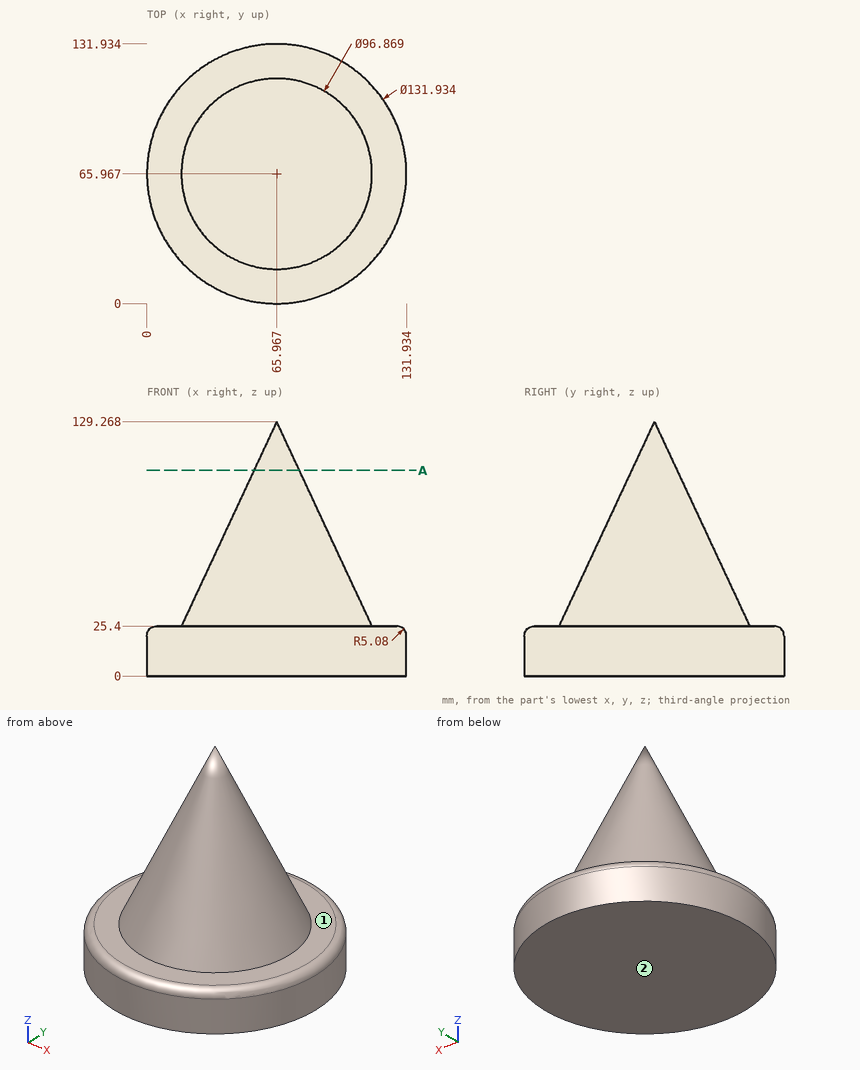
Geometry check sheet. Reference: drawing and pictorial views, mm from the part's lowest x, y, z. A direction names the side the tool comes from. Coordinates: 2 decimals unless noted, no trailing zeros. Loops run counter-clockwise (first coordinate to the right, second up) from the corner with the lowest first, then second, coordinate; pieces in that order, holes last. Notation, with made-up numbers: M -14.5,47 L -5.5,47 A29 cw -5.5,77 Z; hole C 40.25,-2 d8. An arc over 180 degrees is marked long. One line per item, written item: value.
1. Gauge pin test, flat ends, axial feed: P1, Ø10, axis at x = 83, y = 35.5, coming from the -Z side; P2, Ø4, axis at y = 74, z = 89, coming from the +X side; P3, Ø1.5, axis at x = 28.5, y = 32.5, coming from the +Z side; P4, Ø1.5, axis at y = 28.5, z = 37.5, coming from the -X side (1 decimal). Record the tip position at first contact, or that the pin passes through.
Answers follow:
P1: z = 0
P2: x = 84.26
P3: z = 25.4
P4: x = 43.8
2. Material ranges on line 1 along Z through (x, y) = (84, 10); line 2 along X through (y, z) = (64, 9); line 3 along Y through (x, z) = (64.5, 7), recorded low to high. Write a range as from..to.
Answers follow:
line 1: 0..25.4
line 2: 0.03..131.9
line 3: 0.02..131.92
3. Section check A-A on z = 104.5. Record the cut outline in (x, y).
Answers follow:
outline: C 65.97,65.97 d23.1
4. Set-up check for the marked faces 1 and 2: record each of +Z, -Z, +X, -X, +Y, -Y from which the full face is reachable in a straight line by a thin tool's end or side.
Answers follow:
face 1: +Z
face 2: -Z, +X, -X, +Y, -Y
